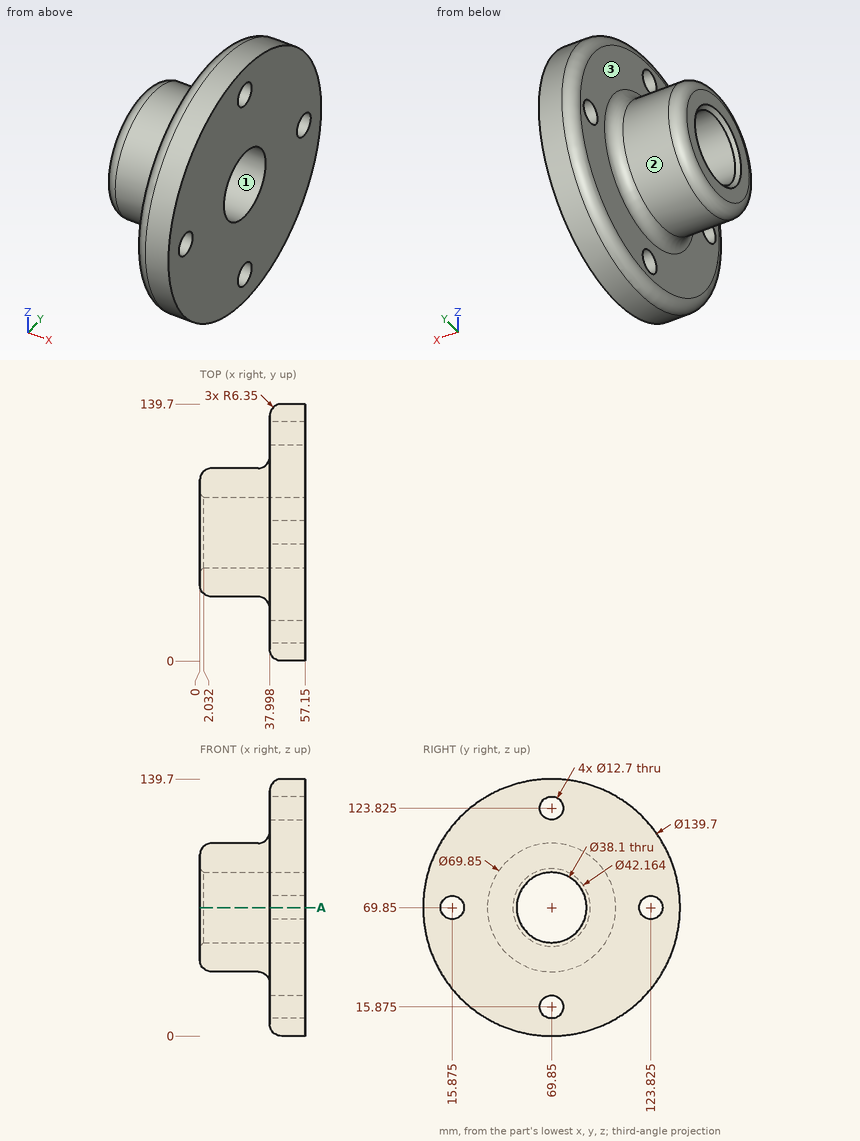
For this review, use the dimensioned drawing (mm, ordinates from the lowest corner) and the shaded views. Give positions to 0.01 mm unless a question says otherwise; leave off trailing zeros.
1. Add section A-A, the plane z = 69.85. State how many separate pieces and enclosed holes the cut face has, then the cut area to 3 significant figures.
Solution:
separate pieces: 4
enclosed holes: 0
area: 2,640 mm2
2. For pin 1 Ø10 at (x, y) = (42.5, 118) entering from -Z (1 decimal); pin 2 Ø7.5 at (y, z) = (15.875, 69.85) entering from -X; pin 3 Ø1 at (x, z) = (8, 38.5) entering from +Y, all flat-tipped, find the tip position at first contact; note any pin that passes through.
Solution:
pin 1: stops at z = 15.1
pin 2: passes through
pin 3: stops at y = 86.22
3. To check wall thickness, follow L1, parallel to Z at x = 48, y = 69 (1 decimal); L2, parallel to X at y = 66, z = 117.5; L3, parallel to Y at x = 39, z = 65 (1 decimal). State the ranges of each line that lie inside material, in increasing order.
Solution:
L1: z = 0 to 9.6, 22.2 to 50.8, 88.9 to 117.5, 130.1 to 139.7
L2: x = 38 to 57.15
L3: y = 3.1 to 11.8, 20 to 51.4, 88.3 to 119.7, 127.9 to 136.6
4. Mouldability with a two-part tool opening along Z and no side actions: class the marked faces 1, 2 and 3 as +Z half, -Z half, draft (parallel to the pull), parting line (faces both ways), or undercut.
Solution:
face 1: undercut
face 2: parting line
face 3: draft
